Geometry check sheet. Reference: the model listing, model coordinates, mm. Face numbers are marked on the shaded views. A direction names the side the tool comes from. Round coordinates to 2 decimals unless told otherwise and drop trailing zeros. Order: outer loops, then holes, each group sorted by start corner. A loop starts at its lowest first (then second) coordinate and runs counter-clockwise, first axis right, second up. Notation, with made-up numbers: (35, 69) - (48, 69) arc R30 ccw to (48, 94) - close; hole circle Ø3 at (-15, -29.5). An arc over 180 degrees is marked (long way). Return JSON: item names as keys, results as strings. Group by question number.
Q1. Tool access check on the marked faces 4, 5 and 6. Record the directions out of +Z, -Z, +X, -X, +Y, -Y that give a thin tool (end or side, any length) a straight path to the whole face; none if there is none.
Q2. Material ranges on line 1 along Y through (x, z) = (0, 2.5); line 2 along Z through (x, y) = (5.25, -1); line 3 along Y through (x, z) = (-4.75, 2.75), recorded low to high.
Q3. Draft check along X on the marked faces 1, 2 and 3. Enter one of: pulls with the +X half, pulls with the -X half, needs draft (parallel to the pull), parting line crosses it, or undercut.
Q4. Sectioned sample at B-B, the plane y = 2.75. Record the cut outline in (x, z).
Q5. Gauge pin test, flat ends, axial feed: pin 1 Ø3 at (x, y) = (-6.5, 8) entering from +Z; pin 2 Ø3 at (y, z) = (8.5, 5) entering from +X; pin 3 Ø5 at (y, z) = (5, 3) entering from +X; pin 4 Ø7 at (x, y) = (0, 0) entering from +Z. Record the tip position at first contact, or that the pin passes through.
Q6. Sectioned sample at A-A, the plane y = 0. Record the cut outline in (x, z), then the cut area to 3 significant figures.
Q7. Sectioned sample at C-C, the plane z = 5. Record the cut outline in (x, y).
```python
from build123d import *

# Parameters (mm, degrees)
F0_R     = 11
F0_R_2   = 1.8
F0_R_3   = 4
F1_DEPTH = 6
F0_R_4   = 3.1
F2_DEPTH = 9
F3_R     = 1.543605
F4_DEPTH = 11.001


with BuildPart() as f1:
    # F0 (on Top) → F1 (new body)
    with BuildSketch(Plane.XY):
        Circle(F0_R)
        with Locations((0, -8)):
            Circle(F0_R_2, mode=Mode.SUBTRACT)
        with Locations((-8, 0)):
            Circle(F0_R_2, mode=Mode.SUBTRACT)
        Circle(F0_R_3, mode=Mode.SUBTRACT)
        with Locations((8, 0)):
            Circle(F0_R_2, mode=Mode.SUBTRACT)
        with Locations((0, 8)):
            Circle(F0_R_2, mode=Mode.SUBTRACT)
    extrude(amount=F1_DEPTH)

    # F0 (on Top) → F2 (join)
    with BuildSketch(Plane.XY):
        Circle(F0_R_3)
        Circle(F0_R_4, mode=Mode.SUBTRACT)
    extrude(amount=F2_DEPTH)

    # F3 (on Right) → F4 (cut, through all)
    with BuildSketch(Plane.YZ):
        with Locations((0, 2.963449)):
            Circle(F3_R)
    extrude(amount=-F4_DEPTH, mode=Mode.SUBTRACT)


solid = f1.part
```
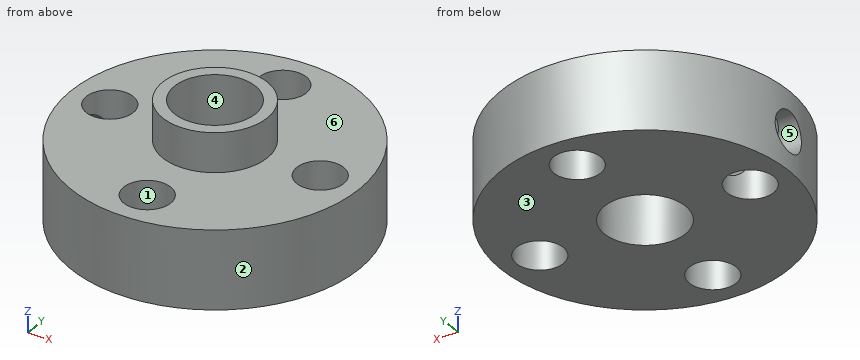
Reply:
{
 "1": {"face 4": "+Z, -Z", "face 5": "-X", "face 6": "+Z"},
 "2": {"line 1": "-11 to -9.8, -6.2 to -3.1, 3.1 to 6.2, 9.8 to 11", "line 2": "0 to 6", "line 3": "-9.92 to -1.53, 1.53 to 9.92"},
 "3": {"face 1": "undercut", "face 2": "parting line crosses it", "face 3": "needs draft"},
 "4": {"outline": "(-10.65, 0) - (-1.43, 0) - (-1.43, 9) - (-2.9, 9) - (-2.9, 6) - (-10.65, 6) - close; (1.43, 0) - (10.65, 0) - (10.65, 6) - (2.9, 6) - (2.9, 9) - (1.43, 9) - close"},
 "5": {"pin 1": "z = 6", "pin 2": "x = 8.49", "pin 3": "x = 10.71", "pin 4": "z = 9"},
 "6": {"outline": "(-11, 0) - (-9.8, 0) - (-9.8, 1.42) - (-11, 1.42) - close; (-11, 4.51) - (-9.8, 4.51) - (-9.8, 6) - (-11, 6) - close; (-6.2, 0) - (-3.1, 0) - (-3.1, 1.42) - (-6.2, 1.42) - close; (-6.2, 4.51) - (-3.1, 4.51) - (-3.1, 9) - (-4, 9) - (-4, 6) - (-6.2, 6) - close; (3.1, 0) - (6.2, 0) - (6.2, 6) - (4, 6) - (4, 9) - (3.1, 9) - close; (9.8, 0) - (11, 0) - (11, 6) - (9.8, 6) - close", "area": "43.7 mm^2"},
 "7": {"outline": "circle Ø22 at (0, 0); hole circle Ø3.6 at (-8, 0); hole circle Ø6.2 at (0, 0); hole circle Ø3.6 at (0, -8); hole circle Ø3.6 at (0, 8); hole circle Ø3.6 at (8, 0)"}
}
